Can you work these out from the drawing? Everything is in mm from the part's minimum corner. Give positions to 0.01 mm unless a question says otherwise; leave off trailing zeros. Order: outer loops, then holes, each group sorted by start corner. A loop starts at its lowest first (then second) coordinate and runs counter-clockwise, first axis right, second up. Notation, with made-up numbers: (-13, 20) - (13, 20) arc R19 ccw to (13, 32) - close; hole circle Ø5 at (61, 70). An arc over 180 degrees is marked (long way). Answer as a JSON object with one key per item and string values.
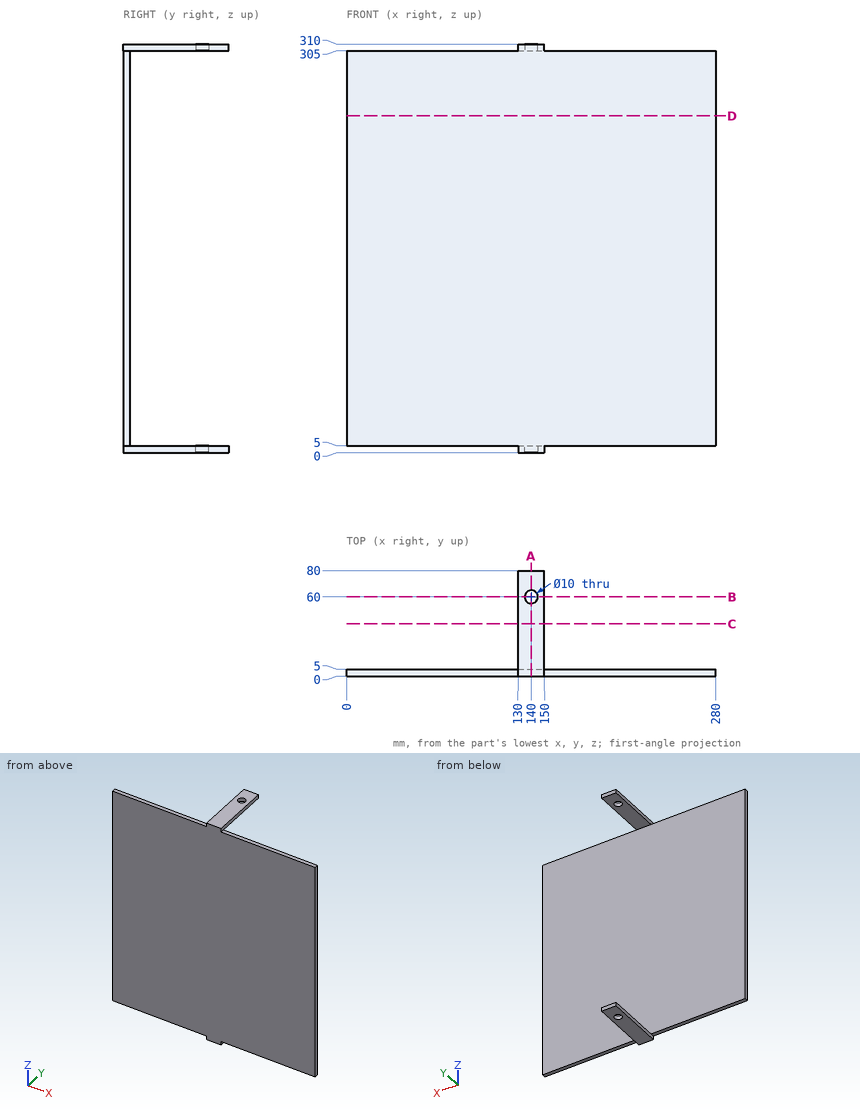
Q1. I'm going to push flat-ended pins straight in: pin 1 Ø4 at (y, z) = (32.5, 308.5) entering from +X; pin 2 Ø5 at (x, z) = (55, 203) entering from +Y; pin 3 Ø9 at (x, y) = (140, 60) entering from -Z; pin 4 Ø4 at (x, y) = (37.5, 1.5) entering from -Z. Where does each tip first touch, or does it pass through?
Recorded:
{"pin 1": "stops at x = 150", "pin 2": "stops at y = 5", "pin 3": "passes through", "pin 4": "stops at z = 5"}
Q2. If we section it at D-D, the plane z = 255.5: Please give me the cut outline in (x, y).
Recorded:
{"outline": "(0, 0) - (280, 0) - (280, 5) - (0, 5) - close"}
Q3. If we section it at C-C, the plane y = 39.5: Please give me the cut outline in (x, z).
Recorded:
{"outline": "(130, 0) - (150, 0) - (150, 5) - (130, 5) - close; (130, 305) - (150, 305) - (150, 310) - (130, 310) - close"}
Q4. If we section it at B-B, the plane y = 60: Please give me the cut outline in (x, z).
Recorded:
{"outline": "(130, 0) - (135, 0) - (135, 5) - (130, 5) - close; (130, 305) - (135, 305) - (135, 310) - (130, 310) - close; (145, 0) - (150, 0) - (150, 5) - (145, 5) - close; (145, 305) - (150, 305) - (150, 310) - (145, 310) - close"}
Q5. If we section it at A-A, the plane x = 140: Please give me the cut outline in (y, z).
Recorded:
{"outline": "(0, 0) - (55, 0) - (55, 5) - (5, 5) - (5, 305) - (55, 305) - (55, 310) - (0, 310) - close; (65, 0) - (80, 0) - (80, 5) - (65, 5) - close; (65, 305) - (80, 305) - (80, 310) - (65, 310) - close"}
Q6. I need wall thicknesses on L1, parallel to Y at x = 140, z = 308; L2, parallel to Z at x = 136, y = 19; L3, parallel to Y at x = 132.5, z = 291. Which ranges of each line are inside material? Lowest first, please.
Recorded:
{"L1": "y = 0 to 55, 65 to 80", "L2": "z = 0 to 5, 305 to 310", "L3": "y = 0 to 5"}
